from build123d import *

# Parameters (mm, degrees)
SKETCH1_W                   = 31.93
SKETCH1_H                   = 30
SKETCH1_W_2                 = 14.88
SKETCH1_H_2                 = 20
BOSS_EXTRUDE1_DEPTH         = 10
SKETCH2_W                   = 10
SKETCH2_H                   = 30
BOSS_EXTRUDE2_DEPTH         = 10
TAP_DRILL_FOR_M5X0_8_TAP1_D = 4.2
FILLET2_R                   = 2
SKETCH5_R                   = 2.5
CUT_EXTRUDE2_DEPTH          = 37.457558887
TAP_DRILL_FOR_M4X0_7_TAP1_D = 3.3
FILLET3_R                   = 2
FILLET4_R                   = 0.5
TAP_DRILL_FOR_M3X0_5_TAP1_D = 2.5
F_4_0_4_DIAMETER_HOLE1_D    = 4


with BuildPart() as part:
    # Sketch1 → Boss-Extrude1 (new body)
    with BuildSketch(Plane(origin=(0, 0, 0), x_dir=(1, 0, 0), z_dir=(0, 1, 0))):
        with Locations((1.475, 0)):
            Rectangle(SKETCH1_W, SKETCH1_H)
        Rectangle(SKETCH1_W_2, SKETCH1_H_2, mode=Mode.SUBTRACT)
    extrude(amount=BOSS_EXTRUDE1_DEPTH)

    # Sketch2 → Boss-Extrude2 (add)
    with BuildSketch(Plane(origin=(0, 10, 0), x_dir=(1, 0, 0), z_dir=(0, 1, 0))):
        with Locations((12.44, 0)):
            Rectangle(SKETCH2_W, SKETCH2_H)
    extrude(amount=BOSS_EXTRUDE2_DEPTH)

    # Tap Drill for M5x0.8 Tap1 (through all)
    with Locations(Plane(origin=(0, 20, 0), x_dir=(1, 0, 0), z_dir=(0, 1, 0))):
        with Locations((12.44, 0)):
            Hole(TAP_DRILL_FOR_M5X0_8_TAP1_D / 2)

    # Fillet2
    fillet2_edges = [part.edges().sort_by_distance(p)[0] for p in [
        (-7.44, 5, -10),
        (-7.44, 5, 10),
        (7.44, 5, 10),
        (7.44, 5, -10),
    ]]
    fillet(fillet2_edges, radius=FILLET2_R)

    # Sketch5 → Cut-Extrude2 (cut, through all)
    with BuildSketch(Plane.XY.offset(-10)):
        with Locations(Location((3.42, 5, 0), (0, 0, 323.900983741))):
            Circle(SKETCH5_R)
    extrude(amount=CUT_EXTRUDE2_DEPTH, mode=Mode.SUBTRACT)

    # Tap Drill for M4x0.7 Tap1 (through all)
    with Locations(Plane.XY.offset(-10)):
        with Locations((3.42, 5)):
            Hole(TAP_DRILL_FOR_M4X0_7_TAP1_D / 2)

    # Fillet3
    fillet3_edges = [part.edges().sort_by_distance(p)[0] for p in [
        (-14.49, 5, -15),
        (-14.49, 5, 15),
    ]]
    fillet(fillet3_edges, radius=FILLET3_R)

    # Fillet4
    fillet4_edges = [part.edges().sort_by_distance(p)[0] for p in [
        (7.44, 15, -15),
        (7.44, 15, 15),
        (17.44, 10, -15),
        (17.44, 10, 15),
    ]]
    fillet(fillet4_edges, radius=FILLET4_R)

    # Tap Drill for M3x0.5 Tap1 (through all)
    with Locations(Plane.ZY.offset(-7.44)):
        with Locations((-11.5, 15), (11.5, 15)):
            Hole(TAP_DRILL_FOR_M3X0_5_TAP1_D / 2)

    # Ø4.0 (4) Diameter Hole1 (through all)
    with Locations(Plane(origin=(0, 10, 0), x_dir=(1, 0, 0), z_dir=(0, 1, 0))):
        with Locations((-10.965, 0)):
            Hole(F_4_0_4_DIAMETER_HOLE1_D / 2)


solid = part.part
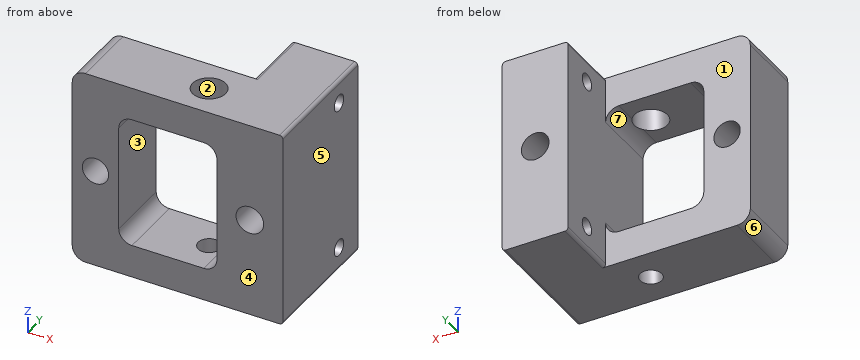
Could you check a few things on this model? Use its own coordinates, in mm. Face numbers are marked on the shaded views. A direction names the side the tool comes from. Coordinates: 2 decimals unless noted, no trailing zeros. Loops run counter-clockwise (first coordinate to the right, second up) from the corner with the lowest first, then second, coordinate; pieces in that order, holes last.
1. Imagine slicing it at B-B (x = 3.42). Please give me the cut outline in (y, z).
2. We'd pull the mould along X, two halves only. Please class the marked faces 4, 5, 6 and 7: released by +X, released by -X, zero draft, split by the parting line, or undercut.
3. For the marked faces 1, 2 and 3, which set-ups out of +Z, -Z, +X, -X, +Y, -Y let a thin tool reach every point of the face, with its end or its side?
4. Imagine slicing it at D-D (y = 5). Please give me the cut outline in (x, z) (3 decimals).
5. I need wall thicknesses on L1, parallel to Z at x = 12, y = 16; L2, parallel to Z at x = -5, y = 3.5; L3, parallel to X at y = 4.5, z = 6. Which ranges of each line are inside material? Lowest first, please.
6. Imagine slicing it at A-A (y = 15). Please give me the cut outline in (x, z).
7. For P1, Ø4, axis at y = 15, z = 11.5, coming from the -X side; P2, Ø10, axis at x = -0.5, z = -10.5, coming from the +Y side, each with a flat end and sliding along its axis, tell me the tip position at first contact or that it passes through.
8. Imagine slicing it at C-C (z = -11.5). Please give me the cut outline in (x, y), and give its area (3 significant figures).
Computed values:
1. outline: (0, -15) - (3.35, -15) - (3.35, -10) - (0, -10) - close; (0, 10) - (2.5, 10) - (2.5, 15) - (0, 15) - close; (6.65, -15) - (10, -15) - (10, -10) - (6.65, -10) - close; (7.5, 10) - (10, 10) - (10, 15) - (7.5, 15) - close
2. face 4: zero draft
2. face 5: released by +X
2. face 6: released by -X
2. face 7: undercut
3. face 1: +Z, -Z, -X, +Y
3. face 2: +Z
3. face 3: +Y, -Y
4. outline: (-14.49, -13) arc R2 ccw to (-12.49, -15) - (1.77, -15) - (1.77, -10) - (-5.44, -10) arc R2 cw to (-7.44, -8) - (-7.44, 8) arc R2 cw to (-5.44, 10) - (0.92, 10) - (0.92, 15) - (-12.49, 15) arc R2 ccw to (-14.49, 13) - close; (5.07, -15) - (16.94, -15) arc R0.5 ccw to (17.44, -14.5) - (17.44, 14.5) arc R0.5 ccw to (16.94, 15) - (5.92, 15) - (5.92, 9.942) arc R2 cw to (7.44, 8) - (7.44, -8) arc R2 cw to (5.92, -9.942) - (5.92, -10) - (5.07, -10) - close; hole circle Ø4 at (-10.965, 0); hole circle Ø4.2 at (12.44, 0)
5. L1: z = -15 to -12.25, -10.75 to -2.05, 2.05 to 10.75, 12.25 to 15
5. L2: z = -15 to -10, 10 to 15
5. L3: x = -14.49 to -7.44, 7.44 to 17.44
6. outline: (7.44, -14.5) arc R0.5 ccw to (7.94, -15) - (16.94, -15) arc R0.5 ccw to (17.44, -14.5) - (17.44, -12.75) - (7.44, -12.75) - close; (7.44, -10.25) - (17.44, -10.25) - (17.44, 10.25) - (7.44, 10.25) - close; (7.44, 12.75) - (17.44, 12.75) - (17.44, 14.5) arc R0.5 ccw to (16.94, 15) - (7.94, 15) arc R0.5 ccw to (7.44, 14.5) - close; hole circle Ø4.2 at (12.44, 0)
7. P1: stops at x = 7.44
7. P2: stops at y = 10
8. outline: (-14.49, 0) - (17.44, 0) - (17.44, 13.75) - (7.44, 13.75) - (7.44, 10) - (-14.49, 10) - close; (7.44, 16.25) - (17.44, 16.25) - (17.44, 20) - (7.44, 20) - close; hole circle Ø3.3 at (3.42, 5)
8. area: 386 mm2
